```python
from build123d import *

# Parameters (mm, degrees)
PAD_DEPTH    = 4
SKETCH001_R  = 1.6
POCKET_DEPTH = 86.001
SKETCH002_R  = 1.6
PAD001_DEPTH = 4
FILLET_R     = 2


with BuildPart() as pocket:
    # Sketch → Pad (new body)
    with BuildSketch(Plane.XY):
        with BuildLine():
            ThreePointArc((24, -6), (32.130235, -2.582329), (38, 4))
            ThreePointArc((38, 4), (47.03758, 36.391617), (45.866557, 70))
            Line((45.866557, 70), (43.866557, 70))
            ThreePointArc((36, 6), (45.123719, 37.362017), (43.866557, 70))
            ThreePointArc((24, -2), (30.615137, 1.077295), (36, 6))
            Line((-12, -2), (24, -2))
            ThreePointArc((-33, 24), (-25.700047, 8.415346), (-12, -2))
            ThreePointArc((-31.852316, 80), (-35.478006, 52.062546), (-33, 24))
            Line((-33.852316, 80), (-31.852316, 80))
            ThreePointArc((-33.852316, 80), (-37.756855, 52.108561), (-36, 24))
            ThreePointArc((-36, 24), (-27.362437, 6.310051), (-12, -6))
            Line((-12, -6), (24, -6))
        make_face()
    extrude(amount=PAD_DEPTH)

    # Sketch001 → Pocket (cut, through all)
    with BuildSketch(Plane.XZ.offset(6)):
        with Locations((-6, 2)):
            Circle(SKETCH001_R)
        with Locations((18, 2)):
            Circle(SKETCH001_R)
    extrude(amount=-POCKET_DEPTH, mode=Mode.SUBTRACT)


with BuildPart() as fillet_body:
    # Sketch002 → Pad001 (new body)
    with BuildSketch(Plane.XY):
        with BuildLine():
            ThreePointArc((-27.855, 26.46), (-24.855, 29.46), (-27.855, 32.46))
            Line((-27.855, 32.46), (-34.855, 32.46))
            Line((-34.855, 32.46), (-34.855, 26.46))
            Line((-34.855, 26.46), (-27.855, 26.46))
        make_face()
        with Locations((-27.855, 29.46)):
            Circle(SKETCH002_R, mode=Mode.SUBTRACT)
        with BuildLine():
            ThreePointArc((40.145, 32.46), (37.145, 29.46), (40.145, 26.46))
            Line((40.145, 26.46), (44.645, 26.46))
            Line((44.645, 32.46), (44.645, 26.46))
            Line((40.145, 32.46), (44.645, 32.46))
        make_face()
        with Locations((40.145, 29.46)):
            Circle(SKETCH002_R, mode=Mode.SUBTRACT)
    extrude(amount=PAD001_DEPTH)

    # Fusion: union Pocket
    add(pocket.part)

    # Fillet
    fillet_edges = [fillet_body.edges().sort_by_distance(p)[0] for p in [
        (-34.397019, 32.46, 2),
        (-33.465486, 26.46, 2),
        (44.39992, 32.46, 2),
        (43.177998, 26.46, 2),
    ]]
    fillet(fillet_edges, radius=FILLET_R)


solid = fillet_body.part
```
The listing builds one solid part. Answer for the finished solid, in the listing's coordinates (mm). A direction names the side the tool comes from. Give positions to 0.01 mm unless a question says otherwise; leave off trailing zeros. Order: outer loops, then holes, each group sorted by start corner. A loop starts at its lowest first (then second) coordinate and runs counter-clockwise, first axis right, second up.
1) Find section C-C on y = 49. Write down the section's boundary in (x, z), then the cut area to 3 significant figures.
Reported:
outline: (-37.84, 0) - (-35.5, 0) - (-35.5, 4) - (-37.84, 4) - close; (45.88, 0) - (47.81, 0) - (47.81, 4) - (45.88, 4) - close
area: 17.1 mm2
2) For faces 1 (the face through (41, 32.46, 2)), 2 (the face through (-37.74, 52.5, 1.97)), 3 (the face through (44.017, 32.954, 1.972)), determine the directions among +Z, -Z, +X, -X, +Y, -Y from which every point of the face is accessible in a straight line to the end or side of a thin tool.
Reported:
face 1: +Z, -Z, +Y
face 2: +Z, -Z, -X
face 3: +Z, -Z
3) Given P1, Ø2, axis at x = 5, z = 2, coming from the +Y side; P2, Ø1.5, axis at y = 15.5, z = 1.5, coming from the +X side; P3, Ø1.3, axis at x = 41, z = 2.5, coming from the +Y side, each flat-ended and moving along its own axis, determine where each tip first touches the part or whether it passes through.
Reported:
P1: stops at y = -2
P2: stops at x = 42.69
P3: stops at y = 32.46
4) Find section B-B on x = -6. Write down the section's boundary in (y, z).
Reported:
outline: (-6, 0) - (-2, 0) - (-2, 0.4) - (-6, 0.4) - close; (-6, 3.6) - (-2, 3.6) - (-2, 4) - (-6, 4) - close
5) Consider line 1 along Y through (x, z) = (7, 0.5); line 2 along X through (y, z) = (35, 2.65); line 3 along X through (y, z) = (17, 3.45). Determine where each line is inside the solid, lowest interval first.
Reported:
line 1: y = -6 to -2
line 2: x = -37.37 to -34.71, 44.81 to 46.86
line 3: x = -33.71 to -30.85, 40.47 to 42.93
6) Find section A-A on z = 2. Give the number of separate pieces and of enclosed holes in the cut face, then the cut area to 3 significant figures.
Reported:
separate pieces: 3
enclosed holes: 2
area: 631 mm2
7) Find section D-D on x = -21.5. Write down the section's boundary in (y, z).
Reported:
outline: (0.25, 0) - (4.03, 0) - (4.03, 4) - (0.25, 4) - close
8) Determine the mould class of faces 4 (the face through (45.865, 51.86, 1.972)), 5 (the face through (5, -4, 4)), 6 (the face through (30.5, 1, 2)), 7 (the face through (-32.614, 25.71, 1.972)) for opening direction Y: pulls with the +Y half, pulls with the -Y half, needs draft (parallel to the pull), parting line crosses it, or undercut.
Reported:
face 4: undercut
face 5: needs draft
face 6: pulls with the +Y half
face 7: undercut
